The model under review builds one solid part; all positions refer to its coordinate system, in mm. Face numbers are marked on the shaded views. A direction names the side the tool comes from. Round coordinates to 2 decimals unless told otherwise and drop trailing zeros. Loops run counter-clockwise (first coordinate to the right, second up) from the corner with the lowest first, then second, coordinate; pieces in that order, holes last. Notation, with made-up numbers: (87.5, 23) -> (137.5, 23) arc R25 cw to (137.5, 57) -> close; hole circle Ø7 at (-25, 75). An arc over 180 degrees is marked (long way). Use a Markdown table: item, result. Add a question column.
1) Mouldability with a two-part tool opening along X and no side actions: class the marked faces 4, 5 and 6 as released by +X, released by -X, zero draft, split by the parting line, or undercut.
2) For the marked faces 1, 2 and 3, list the 3-axis set-ups (+Z, -Z, +X, -X, +Y, -Y) from which the entire face can be reached by the end or side of a thin tool; tool diameter is ignored.
3) Consider section C-C on y = 22.5. Give the boundary of the cut face in (x, z), plus the area to 4 significant figures.
4) Consider section B-B on x = 31. Give the boundary of the cut face in (y, z).
5) Insertion check: pin 1 (4 mm diameter, centred on x = 69.5, z = 6, fed in from +Y); pin 2 (3 mm diameter, centred on x = 98.5, z = 27.5, fed in from -Y); pin 3 (3 mm diameter, centred on x = 58.5, y = 12.5, fed in from +Z). Each pin has a flat end and moves straight along its axis. Give the tip position at first contact, or say it passes through.
6) Consider section A-A on y = 5. Give the boundary of the cut face in (x, z), plus the area to 4 significant figures.
7) Wall thickness on probe 1 along Y at (x, z) = (15.5, 7.5); probe 2 along X at (y, z) = (23.5, 19); probe 3 along Z at (x, y) = (105, 26.5): over which ranges is each line inside the solid? List them lowest first.
8) Consider section D-D on x = 82.5. Give the boundary of the cut face in (y, z).
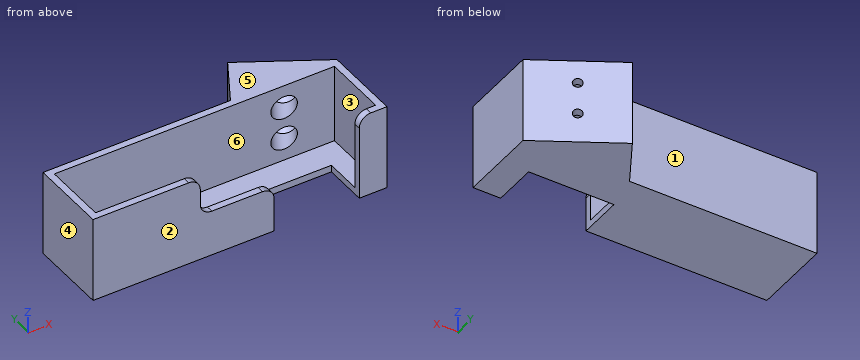
from build123d import *

# Parameters (mm, degrees)
F1_DEPTH = 34
F2_DEPTH = 3
F3_W     = 32
F3_H     = 17
F4_DEPTH = 3
F6_D     = 4
F9_D     = 10
F9_DEPTH = 6.6
F9_START = 8.6756443
F9_TIP   = 3.0043030951
F10_R    = 5


with BuildPart() as f1:
    # F0 (on Top) → F1 (new body)
    with BuildSketch(Plane.XY):
        Polygon((75.5, 0), (0, 0), (0, 28), (121.5, 28), (121.5, 0), (112.5, 0), (112.5, -3), (124.5, -3), (124.5, 31), (89.8589838486, 51), (78.3119784648, 31), (-3, 31), (-3, -3), (75.5, -3), align=None)
    extrude(amount=F1_DEPTH)

    # F0 (on Top) → F2 (join)
    with BuildSketch(Plane.XY):
        Polygon((0, 28), (0, 0), (75.5, 0), (75.5, 16), (112.5, 16), (112.5, 0), (121.5, 0), (121.5, 28), align=None)
        Polygon((75.5, 0), (0, 0), (0, 28), (121.5, 28), (121.5, 0), (112.5, 0), (112.5, -3), (124.5, -3), (124.5, 31), (89.8589838486, 51), (78.3119784648, 31), (-3, 31), (-3, -3), (75.5, -3), align=None)
    extrude(amount=-F2_DEPTH)

    # F3 (on face) → F4 (cut, through all)
    with BuildSketch(Plane.XZ.offset(3)):
        with Locations((59.5, 25.5)):
            Rectangle(F3_W, F3_H)
    extrude(amount=-F4_DEPTH, mode=Mode.SUBTRACT)

    # F6 (through all)
    with Locations(Plane(origin=(44.5483937587, 77.1600813856, 0), x_dir=(-0.8660254038, 0.5, 0), z_dir=(0.5, 0.8660254038, 0))):
        with Locations((-72.3201627712, 24), (-72.3201627712, 10)):
            Hole(F6_D / 2)

    # F9
    # its depths count from where the whole tool has entered the part; down to there all is cleared
    with Locations(Plane(origin=(34.1483937587, 59.1467529869, 0), x_dir=(-0.8660254038, 0.5, 0), z_dir=(-0.5, -0.8660254038, 0))):
        with Locations((-72.3201627712, -24), (-72.3201627712, -10)):
            Hole(F9_D / 2, depth=F9_START)
    with Locations(Plane(origin=(34.1483937587, 59.1467529869, 0), x_dir=(-0.8660254038, 0.5, 0), z_dir=(-0.5, -0.8660254038, 0)).offset(-F9_START)):
        with Locations((-72.3201627712, -24), (-72.3201627712, -10)):
            Hole(F9_D / 2, depth=F9_DEPTH)
            with Locations((0, 0, -(F9_DEPTH + F9_TIP / 2))):  # 118° drill point
                Cone(0, F9_D / 2, F9_TIP, mode=Mode.SUBTRACT)

    # F10
    f10_edges = [f1.edges().sort_by_distance(p)[0] for p in [
        (112.5, -1.5, 34),
        (43.5, -1.5, 34),
        (75.5, -1.5, 17),
        (43.5, -1.5, 17),
    ]]
    fillet(f10_edges, radius=F10_R)


solid = f1.part
Result set:
| question | item | result |
|---|---|---|
| 1 | face 4 | released by -X |
| 1 | face 5 | zero draft |
| 1 | face 6 | undercut |
| 2 | face 1 | +Z, -Z, -X, +Y |
| 2 | face 2 | +Z, -Z, +X, -X, -Y |
| 2 | face 3 | +Z |
| 3 | outline | (-3, -3) -> (124.5, -3) -> (124.5, 34) -> (121.5, 34) -> (121.5, 0) -> (0, 0) -> (0, 34) -> (-3, 34) -> close |
| 3 | area | 586.5 mm2 |
| 4 | outline | (-3, -3) -> (31, -3) -> (31, 34) -> (28, 34) -> (28, 0) -> (0, 0) -> (0, 34) -> (-3, 34) -> close |
| 5 | pin 1 | y = 31 |
| 5 | pin 2 | y = 28 |
| 5 | pin 3 | z = 0 |
| 6 | outline | (-3, -3) -> (75.5, -3) -> (75.5, 0) -> (0, 0) -> (0, 34) -> (-3, 34) -> close; (112.5, -3) -> (124.5, -3) -> (124.5, 34) -> (121.5, 34) -> (121.5, 0) -> (112.5, 0) -> close |
| 6 | area | 475.5 mm2 |
| 7 | probe 1 | -3 to 0, 28 to 31 |
| 7 | probe 2 | -3 to 0, 121.5 to 124.5 |
| 7 | probe 3 | -3 to 0 |
| 8 | outline | (16, -3) -> (38.25, -3) -> (38.25, 34) -> (28, 34) -> (28, 0) -> (16, 0) -> close |
